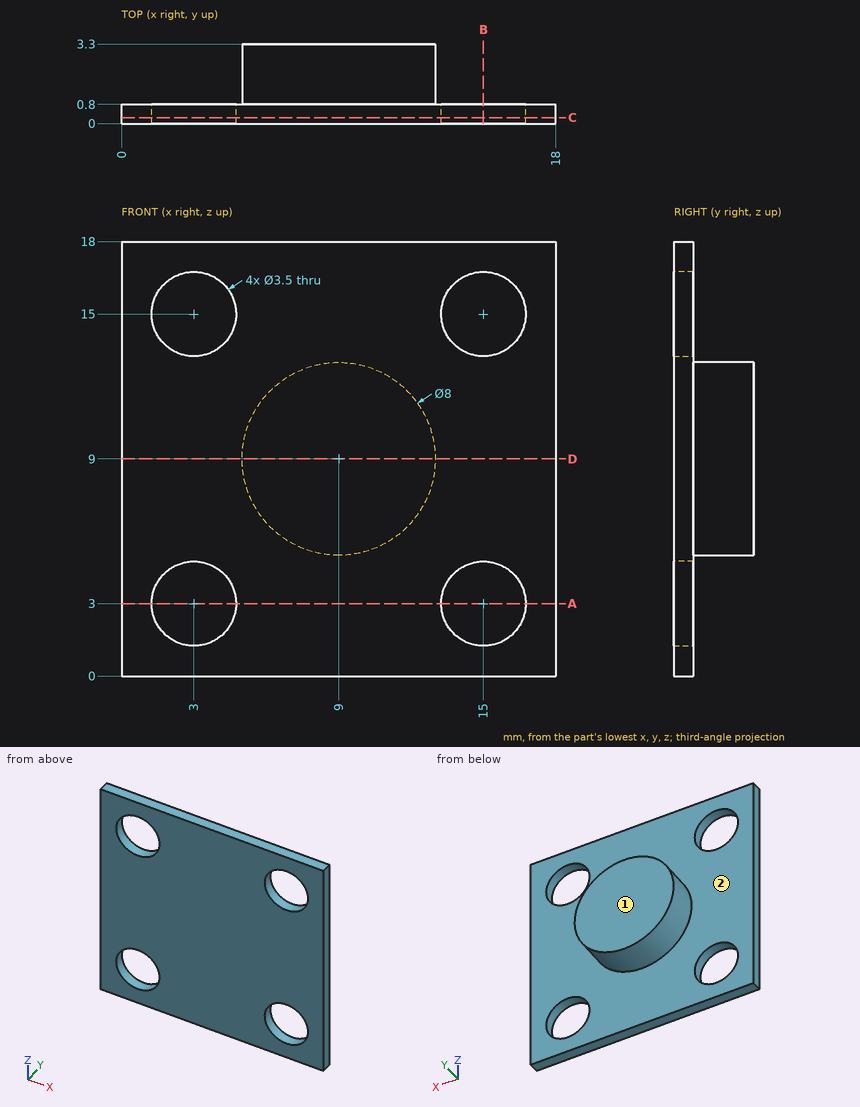
Source: three-view drawing plus pictorial views. Frame: mm from the lowest corner of the part. A direction names the side the tool comes from. Round coordinates to 2 decimals unless told otherwise and drop trailing zeros. Write each loop counter-clockwise with the first axis right and the second up, starting at its lowest first coordinate (ties: lowest second). Pieces come first, ordered by that corner, then holes. Notation, with made-up numbers: M -7,-28 L 22,-28 A21 cw 22,-2 Z; hole C 74,86 d9. An arc over 180 degrees is marked long. Use CSV: the item, a comma, the result in double quotes. Start each with the question number.
Q1. Line query: line 1 (X direction, y = 0.65, z = 15); line 2 (Y direction, x = 6.25, z = 4.5); line 3 (X direction, y = 2.2, z = 7.25). Output: solid intervals per line, ascending. Write a range as from..to.
Q2. Cut plane B-B on x = 15. Output: boundary loops of the cut face in (y, z).
Q3. Cut plane A-A on z = 3. Output: boundary loops of the cut face in (x, y).
Q4. Cut plane D-D on z = 9. Output: boundary loops of the cut face in (x, y).
Q5. Cut plane C-C on y = 0.25. Output: boundary loops of the cut face in (x, z).
Q6. Access query for the marked faces 1 and 2. Directions: +Z, -Z, +X, -X, +Y, -Y. A direction counts if a zero-diameter tool reaches every point of the face in a straight line with its end or side. Return the directions, or none.
Q7. First-contact query: P1, Ø2, axis at x = 15, z = 3, coming from the -Y side; P2, Ø1, axis at y = 3, z = 13, coming from the -X side; P3, Ø3, axis at x = 15.5, z = 7, coming from the +Y side. Flat tips, straight axial feed; report the tip coordinate or a pass-through.
Results found:
1,line 1,"0..1.25, 4.75..13.25, 16.75..18"
1,line 2,"0..0.8"
1,line 3,"5.4..12.6"
2,outline,"M 0,0 L 0.8,0 L 0.8,1.25 L 0,1.25 Z; M 0,4.75 L 0.8,4.75 L 0.8,13.25 L 0,13.25 Z; M 0,16.75 L 0.8,16.75 L 0.8,18 L 0,18 Z"
3,outline,"M 0,0 L 1.25,0 L 1.25,0.8 L 0,0.8 Z; M 4.75,0 L 13.25,0 L 13.25,0.8 L 4.75,0.8 Z; M 16.75,0 L 18,0 L 18,0.8 L 16.75,0.8 Z"
4,outline,"M 0,0 L 18,0 L 18,0.8 L 13,0.8 L 13,3.3 L 5,3.3 L 5,0.8 L 0,0.8 Z"
5,outline,"M 0,0 L 18,0 L 18,18 L 0,18 Z; hole C 3,3 d3.5; hole C 3,15 d3.5; hole C 15,3 d3.5; hole C 15,15 d3.5"
6,face 1,"+Z, -Z, +X, -X, +Y"
6,face 2,"+Y"
7,P1,"through"
7,P2,"x = 7.06"
7,P3,"y = 0.8"
